Autodesk Inventor part; units mm, degrees
ref_plane "YZ Plane" through (0, 0, 0) normal (1, 0, 0) x (0, 1, 0)
ref_plane "XZ Plane" through (0, 0, 0) normal (0, 1, 0) x (-1, 0, 0)
ref_plane "XY Plane" through (0, 0, 0) normal (0, 0, 1) x (1, 0, 0)
sketch "Sketch1" plane through (0, 0, 0) normal (0, 1, 0) x (-1, 0, 0)
  line L0 (0, 0) -> (-90, 0)
  line L1 (-90, 0) -> (-90, -90)
  line L2 (-90, -90) -> (0, -90)
  line L3 (0, -90) -> (0, 0)
  dimension "d0" = 90
  dimension "d1" = 90
extrude "Extrusion1" add sketch "Sketch1" along normal blind 88.9
sketch "Sketch2" plane through (90, 0, 0) normal (1, 0, 0) x (0, 0, -1)
  line L0 (0, 0) -> (90, 0)
  line L1 (90, 0) -> (90, 88.9)
  line L2 (0, 88.9) -> (90, 88.9)
  line L3 (0, 0) -> (0, 88.9)
  line L4 (0, 88.9) -> (1.6, 88.9)
  line L5 (0, 88.9) -> (90, 88.9)
  line L6 (1.6, 88.9) -> (6.2, 88.9)
  line L7 (6.2, 88.9) -> (7.8, 88.9)
  line L8 (7.8, 88.9) -> (7.8, 8.402)
  line L9 (6.2, 88.9) -> (6.2, 8.402)
  line L10 (1.6, 88.9) -> (1.6, 8.402)
  line L11 (1.6, 8.402) -> (6.2, 8.402)
  line L12 (90, 88.9) -> (88.4, 88.9)
  line L13 (88.4, 88.9) -> (88.4, 8.402)
  line L14 (88.4, 8.402) -> (83.8, 8.402)
  line L15 (83.8, 8.402) -> (83.8, 88.9)
  dimension "d4" = 1.6
  dimension "d5" = 4.6
  dimension "d6" = 1.6
  dimension "d7" = 1.6
  dimension "d8" = 4.6
extrude "Extrusion2" cut sketch "Sketch2" against normal blind 127 contours L2 L9 L11 L10 | L13 L14 L15 L2
sketch "Sketch3" plane through (90, 0, 0) normal (1, 0, 0) x (0, 0, -1)
  line L0 (1.6, 8.402) -> (1.6, 88.9)
  line L1 (0, 88.9) -> (1.6, 88.9)
  line L2 (0, 0) -> (0, 88.9)
  line L3 (0, 0) -> (90, 0)
  line L4 (90, 0) -> (90, 88.9)
  line L5 (88.4, 88.9) -> (90, 88.9)
  line L6 (88.4, 88.9) -> (88.4, 8.402)
  line L7 (88.4, 8.402) -> (83.8, 8.402)
  line L8 (83.8, 8.402) -> (83.8, 88.9)
  line L9 (6.2, 88.9) -> (83.8, 88.9)
  line L10 (6.2, 88.9) -> (6.2, 8.402)
  line L11 (6.2, 8.402) -> (1.6, 8.402)
sketch "Sketch5" plane through (90, 0, 0) normal (1, 0, 0) x (0, 0, -1)
  line L0 (-0.0003, 88.9) -> (90, 88.9)
  line L1 (90, 88.9) -> (90, 38.1)
  line L2 (90, 38.1) -> (-0.0003, 38.1)
  line L3 (-0.0003, 38.1) -> (-0.0003, 88.9)
  point P0 (0, 0)
  dimension "d24" = 50.8
extrude "Extrusion3" cut sketch "Sketch5" against normal blind 111.125
sketch "Sketch6" plane through (90, 0, 0) normal (1, 0, 0) x (0, 0, -1)
  line L0 (1.6, 38.1) -> (0, 38.1)
  line L1 (0, 0) -> (0, 38.1)
  line L2 (0, 0) -> (90, 0)
  line L3 (90, 0) -> (90, 38.1)
  line L4 (90, 38.1) -> (88.4, 38.1)
  line L5 (88.4, 38.1) -> (88.4, 8.402)
  line L6 (88.4, 8.402) -> (83.8, 8.402)
  line L7 (83.8, 8.402) -> (83.8, 38.1)
  line L8 (83.8, 38.1) -> (6.2, 38.1)
  line L9 (6.2, 38.1) -> (6.2, 8.402)
  line L10 (6.2, 8.402) -> (1.6, 8.402)
  line L11 (1.6, 8.402) -> (1.6, 38.1)
  line L12 (6.2, 38.1) -> (6.2, 8.402)
  line L13 (6.2, 8.402) -> (10.01, 8.402)
  line L14 (10.01, 8.402) -> (10.01, 38.1)
  line L15 (10.01, 38.1) -> (6.2, 38.1)
  line L16 (10.01, 38.1) -> (10.01, 8.402)
  line L17 (10.01, 8.402) -> (22.71, 8.402)
  line L18 (22.71, 8.402) -> (22.71, 38.1)
  line L19 (22.71, 38.1) -> (10.01, 38.1)
  line L20 (22.71, 38.1) -> (22.71, 8.402)
  line L21 (22.71, 8.402) -> (26.52, 8.402)
  line L22 (26.52, 8.402) -> (26.52, 38.1)
  line L23 (26.52, 38.1) -> (22.71, 38.1)
  line L24 (26.52, 38.1) -> (26.52, 8.402)
  line L25 (26.52, 8.402) -> (30.33, 8.402)
  line L26 (30.33, 8.402) -> (30.33, 38.1)
  line L27 (30.33, 38.1) -> (26.52, 38.1)
  line L28 (30.33, 38.1) -> (30.33, 8.402)
  line L29 (30.33, 8.402) -> (34.14, 8.402)
  line L30 (34.14, 8.402) -> (34.14, 38.1)
  line L31 (34.14, 38.1) -> (30.33, 38.1)
  line L32 (83.8, 38.1) -> (83.8, 8.402)
  line L33 (83.8, 8.402) -> (79.99, 8.402)
  line L34 (79.99, 8.402) -> (79.99, 38.1)
  line L35 (79.99, 38.1) -> (83.8, 38.1)
  line L36 (79.99, 38.1) -> (79.99, 8.402)
  line L37 (79.99, 8.402) -> (67.29, 8.402)
  line L38 (67.29, 8.402) -> (67.29, 38.1)
  line L39 (67.29, 38.1) -> (79.99, 38.1)
  line L40 (67.29, 38.1) -> (67.29, 8.402)
  line L41 (67.29, 8.402) -> (63.48, 8.402)
  line L42 (63.48, 8.402) -> (63.48, 38.1)
  line L43 (63.48, 38.1) -> (67.29, 38.1)
  line L44 (63.48, 38.1) -> (63.48, 8.402)
  line L45 (63.48, 8.402) -> (59.67, 8.402)
  line L46 (59.67, 8.402) -> (59.67, 38.1)
  line L47 (59.67, 38.1) -> (63.48, 38.1)
  line L48 (59.67, 38.1) -> (59.67, 8.402)
  line L49 (59.67, 8.402) -> (55.86, 8.402)
  line L50 (55.86, 8.402) -> (55.86, 38.1)
  line L51 (55.86, 38.1) -> (59.67, 38.1)
  line L52 (55.86, 38.1) -> (55.86, 8.402)
  line L53 (55.86, 8.402) -> (48.24, 8.402)
  line L54 (48.24, 8.402) -> (48.24, 38.1)
  line L55 (48.24, 38.1) -> (55.86, 38.1)
  line L56 (34.14, 38.1) -> (34.14, 8.402)
  line L57 (34.14, 8.402) -> (41.76, 8.402)
  line L58 (41.76, 8.402) -> (41.76, 38.1)
  line L59 (41.76, 38.1) -> (34.14, 38.1)
  dimension "d27" = 3.81
  dimension "d28" = 12.7
  dimension "d29" = 3.81
  dimension "d30" = 3.81
  dimension "d31" = 3.81
  dimension "d32" = 3.81
  dimension "d33" = 12.7
  dimension "d34" = 3.81
  dimension "d35" = 3.81
  dimension "d36" = 3.81
  dimension "d37" = 7.62
  dimension "d38" = 7.62
extrude "Extrusion4" cut sketch "Sketch6" against normal blind 111.125 contours L14 L8 L18 L17 | L22 L8 L26 L25 | L30 L8 L58 L57 | L37 L38 L8 L34 | L45 L46 L8 L42 | L8 L50 L53 L54
properties part number "HeatSink" material "Aluminum 6061"
Work out the finished part from the listing and answer in its coordinate system (mm). A direction names the side the tool comes from. Give positions to 0.01 mm unless a question says otherwise; leave off trailing zeros. Order: outer loops, then holes, each group sorted by start corner. A loop starts at its lowest first (then second) coordinate and runs counter-clockwise, first axis right, second up. Notation, with made-up numbers: (4.25, 82) -> (14.25, 82) arc R24 ccw to (14.25, 106) -> close; hole circle Ø9 at (44, -20.75). An arc over 180 degrees is marked (long way). Answer as a JSON object with one key per item and string values. Group by question number.
1. Consider line 1 along Y through (x, z) = (33, -51.5). Determine where the line is inside the solid, lowest interval first. Write a range as [from, to].
2. The mould has two halves that part along Z. Classify faces 3 (the flat face through (0, 15, -46)), 4 (the flat face through (46, 23, -59.67)): released by +Z, released by -Z, zero draft, split by the parting line, or undercut.
3. Section A-A on y = 36.5 is taken. Count the separate pieces of the cut face and the enclosed holes in it, plus the area to 3 significant figures.
4. Section B-B on z = -74.5 is taken. Determine the outline of the cut face in (x, y).
5. A flat-ended cylindrical pin translates along its axis: pin 1 Ø1.9 at (x, z) = (52.5, -28) entering from +Y. Find the tip coordinate at first contact, or state that the pin passes through.
6. A tool of negligible diameter and unlimited length cuts with its end or side. For faces 1 (the flat face through (46, 0, -44)), 2 (the flat face through (46, 23, -30.33)), from which of +Z, -Z, +X, -X, +Y, -Y can it reach the whole face along a straight path? Write none if from no direction.
Result sheet:
{
 "1": {"line 1": "y = [0, 8.4]"},
 "2": {"face 3": "zero draft", "face 4": "undercut"},
 "3": {"separate pieces": "9", "enclosed holes": "0", "area": "2,930 mm^2"},
 "4": {"outline": "(0, 0) -> (90, 0) -> (90, 8.4) -> (0, 8.4) -> close"},
 "5": {"pin 1": "stops at y = 8.4"},
 "6": {"face 1": "+Z, -Z, +X, -X, -Y", "face 2": "+X, -X, +Y"}
}
